Build history of the part. All positions in model axes, mm. A direction names the side the tool comes from. Give positions to 0.01 mm unless a question says otherwise; leave off trailing zeros. Order: outer loops, then holes, each group sorted by start corner. A loop starts at its lowest first (then second) coordinate and runs counter-clockwise, first axis right, second up. Notation, with made-up numbers: M 49,-10 L 95,-10 A34 ccw 95,21 Z; hole C 66.5,-24.75 d1. An arc over 180 degrees is marked long. Answer as CSV lines item,"result".
from build123d import *

# Parameters (mm, degrees)
SKETCH_3_R           = 1.72
CUT_EXTRUDE_1_DEPTH  = 20.918584287
SKETCH_5_R           = 1.45
CUT_EXTRUDE_2_DEPTH  = 20.918584287
SKETCH_6_OUTSIDE_W   = 31.9
SKETCH_6_OUTSIDE_H   = 31.9
SKETCH_6_OUTSIDE_W_2 = 15
SKETCH_6_OUTSIDE_H_2 = 23
CUT_EXTRUDE_3_DEPTH  = 20.918584287


with BuildPart() as part:
    # 草图2 → 旋转1 (revolve)
    with BuildSketch(Plane.XY, mode=Mode.PRIVATE) as revolve_1_sk:
        Polygon((-5.75, 0), (-5.75, 5), (2.25, 5), (2.25, 11.5), (5.75, 11.5), (5.75, 0), align=None)
    revolve(revolve_1_sk.sketch.rotate(Axis((5.75, 0, 0), (-1, 0, 0)), 90), axis=Axis((5.75, 0, 0), (-1, 0, 0)))

    # 草图3 → 切除-拉伸1 (cut, through all)
    with BuildSketch(Plane.ZY.offset(5.75)):
        with Locations(Location((0, 0, 0), (0, 0, 270))):
            Circle(SKETCH_3_R)
    extrude(amount=-CUT_EXTRUDE_1_DEPTH, mode=Mode.SUBTRACT)

    # 草图5 → 切除-拉伸2 (cut, through all)
    with BuildSketch(Plane(origin=(5.75, 0, 0), x_dir=(0, 0, -1), z_dir=(1, 0, 0))):
        with Locations((-3.75, 6.495190528)):
            Circle(SKETCH_5_R)
        with Locations((3.75, 6.495190528)):
            Circle(SKETCH_5_R)
        with Locations((-3.75, -6.495190528)):
            Circle(SKETCH_5_R)
        with Locations((3.75, -6.495190528)):
            Circle(SKETCH_5_R)
    extrude(amount=-CUT_EXTRUDE_2_DEPTH, mode=Mode.SUBTRACT)

    # 草图6 outside → 切除-拉伸3 (cut, through all)
    with BuildSketch(Plane(origin=(5.75, 0, 0), x_dir=(0, 0, -1), z_dir=(1, 0, 0))):
        Rectangle(SKETCH_6_OUTSIDE_W, SKETCH_6_OUTSIDE_H)
        Rectangle(SKETCH_6_OUTSIDE_W_2, SKETCH_6_OUTSIDE_H_2, mode=Mode.SUBTRACT)
    extrude(amount=-CUT_EXTRUDE_3_DEPTH, mode=Mode.SUBTRACT)


solid = part.part
Item 1: 3-axis set-ups, long thin cutter, end or side, ignore diameter. For faces 5 (the flat face through (5.75, 0, 2)), 6 (the cylindrical face through (-2, 0, 5)): which of +Z, -Z, +X, -X, +Y, -Y reach the whole face in a straight line?
Geometry says:
face 5,"+Z, -Z, +X, +Y, -Y"
face 6,"-X"
Item 2: Band-saw the part on C-C (z = 2.75). Give the cut face in (x, y).
Geometry says:
outline,"M -5.75,-4.18 L 2.25,-4.18 L 2.25,-5.45 L 5.75,-5.45 L 5.75,5.45 L 2.25,5.45 L 2.25,4.18 L -5.75,4.18 Z; M 2.25,-11.17 L 5.75,-11.17 L 5.75,-7.55 L 2.25,-7.55 Z; M 2.25,7.55 L 5.75,7.55 L 5.75,11.17 L 2.25,11.17 Z"
Item 3: Band-saw the part on D-D (x = -3.5). Give the cut face in (y, z).
Geometry says:
outline,"C 0,0 d10; hole C 0,0 d3.44"
Item 4: Band-saw the part on B-B (y = 0). Give the cut face in (x, z).
Geometry says:
outline,"M -5.75,-5 L 2.25,-5 L 2.25,-7.5 L 5.75,-7.5 L 5.75,-1.72 L -5.75,-1.72 Z; M -5.75,1.72 L 5.75,1.72 L 5.75,7.5 L 2.25,7.5 L 2.25,5 L -5.75,5 Z"
Item 5: Band-saw the part on A-A (z = 0). Give the cut face in (x, y).
Geometry says:
outline,"M -5.75,-5 L 2.25,-5 L 2.25,-11.5 L 5.75,-11.5 L 5.75,-1.72 L -5.75,-1.72 Z; M -5.75,1.72 L 5.75,1.72 L 5.75,11.5 L 2.25,11.5 L 2.25,5 L -5.75,5 Z"
Item 6: Drop flat-ended pins along their axis: pin 1 (6 mm diameter, centred on x = -1.5, y = -7, fed in from +Z); pin 2 (4.5 mm diameter, centred on y = 6.5, z = -3.75, fed in from -X); pin 3 (2.5 mm diameter, centred on y = -6.5, z = 3.75, fed in from -X). Give the stop position or say it passes through.
Geometry says:
pin 1,"stops at z = 3"
pin 2,"stops at x = 2.25"
pin 3,"passes through"
Item 7: Probe line 1 along Y through (x, z) = (5.25, 3); line 2 along Y through (x, z) = (4, -3.75); line 3 along X through (y, z) = (-9, -3.25). List the from-to ranges inside material, lowest first. Write a range as from..to.
Geometry says:
line 1,"y = -11.1..-7.74, -5.25..5.25, 7.74..11.1"
line 2,"y = -10.87..-7.95, -5.05..5.05, 7.95..10.87"
line 3,"x = 2.25..5.75"
Item 8: Pull direction Y, two halves, no side cores. Call faces 1 (the cylindrical face through (4.02, -7.38, -2.6)), 2 (the flat face through (2.25, 5, -2)), 3 (the cylindrical face through (4, -11.5, -0.1)), 4 (the cylindrical face through (4.02, -7.38, 4.9)): released by +Y, released by -Y, zero draft, split by the parting line, or undercut.
Geometry says:
face 1,"undercut"
face 2,"zero draft"
face 3,"released by -Y"
face 4,"undercut"
